Work out the finished part from the listing and answer in its coordinate system (mm). Give positions to 0.01 mm unless a question says otherwise; leave off trailing zeros. Order: outer loops, then holes, each group sorted by start corner. A loop starts at its lowest first (then second) coordinate and runs counter-clockwise, first axis right, second up. Notation, with made-up numbers: (18.25, -8.75) -> (65.25, -8.75) arc R30 ccw to (65.25, 25.25) -> close; hole circle Ø10 at (26, 36). An arc over 180 degrees is marked (long way). Use a Markdown table: item, result. Add a question column.
```python
from build123d import *

# Parameters (mm, degrees)
F0_W     = 800
F0_H     = 95
F1_DEPTH = 8
F2_SIZE  = 30
F4_D     = 10


with BuildPart() as f1:
    # F0 (on Front) → F1 (new body, symmetric)
    with BuildSketch(Plane.XZ):
        Rectangle(F0_W, F0_H)
    extrude(amount=F1_DEPTH, both=True)

    # F2
    f2_edges = [f1.edges().sort_by_distance(p)[0] for p in [
        (-400, 0, -47.5),
        (-400, 0, 47.5),
        (400, 0, -47.5),
        (400, 0, 47.5),
    ]]
    chamfer(f2_edges, length=F2_SIZE)

    # F4 (through all)
    with Locations(Plane.XZ.offset(8)):
        with Locations((0, 0), (300, 0), (-300, 0)):
            Hole(F4_D / 2)


solid = f1.part
```
1) The part is cut by section C-C, the plane z = 36.5. Determine the outline of the cut face in (x, y), then the cut area to 3 significant figures.
2) Straight lines are drawn through the part: line 1 (Z direction, x = 0, y = 3.5); line 2 (X direction, y = -5.25, z = 34.5); line 3 (X direction, y = -1.5, z = -23). For each, find the intervals that lie inside material, in ascending order.
3) The part is cut by section B-B, the plane z = -32. Determine the outline of the cut face in (x, y), then the cut area to 3 significant figures.
4) The part is cut by section A-A, the plane y = 4. Determine the outline of the cut face in (x, z), then the cut area to 3 significant figures.
5) A flat-ended cylindrical pin translates along its axis: pin 1 (4 mm diameter, centred on y = 0, z = 20.5, fed in from +X). Find the tip coordinate at first contact, or state that the pin passes through.
A:
| question | item | result |
|---|---|---|
| 1 | outline | (-381, -8) -> (381, -8) -> (381, 8) -> (-381, 8) -> close |
| 1 | area | 12,200 mm^2 |
| 2 | line 1 | -47.5 to -5, 5 to 47.5 |
| 2 | line 2 | -383 to 383 |
| 2 | line 3 | -394.5 to 394.5 |
| 3 | outline | (-385.5, -8) -> (385.5, -8) -> (385.5, 8) -> (-385.5, 8) -> close |
| 3 | area | 12,300 mm^2 |
| 4 | outline | (-400, -17.5) -> (-370, -47.5) -> (370, -47.5) -> (400, -17.5) -> (400, 17.5) -> (370, 47.5) -> (-370, 47.5) -> (-400, 17.5) -> close; hole circle Ø10 at (-300, 0); hole circle Ø10 at (0, 0); hole circle Ø10 at (300, 0) |
| 4 | area | 74,000 mm^2 |
| 5 | pin 1 | x = 399 |
